Verification items for the finished model (mm, model axes). A direction names the side the tool comes from. Round coordinates to 2 decimals unless told otherwise and drop trailing zeros. Order: outer loops, then holes, each group sorted by start corner. A loop starts at its lowest first (then second) coordinate and runs counter-clockwise, first axis right, second up. Notation, with made-up numbers: (-21, -20.5) -> (-3, -20.5) arc R35 cw to (-3, 17.5) -> close; hole circle Ø2 at (-1, 7). An arc over 180 degrees is marked (long way). Return JSON: item names as keys, results as strings. Group by question number.
1) Section check D-D on z = -291.8. State how many separate pieces and enclosed holes the cut face has, plus the area to 3 significant figures.
2) Tool access check on faces 1 (the flat face through (612.722, -14, -282)), 2 (the cylindrical face through (602.03, -28.09, -291.98)), 3 (the flat face through (597, -20, -292)), 4 (the flat face through (610, -20, -260)), 5 (the flat face through (595.962, -41.363, -306.052)). Record the directions out of +Z, -Z, +X, -X, +Y, -Y that give a thin tool (end or side, any length) a straight path to the whole face; none if there is none.
3) Depth check by flat-ended pin: pin 1 (17 mm diameter, centred on x = 597, z = -287.5, fed in from +Y); pin 2 (13 mm diameter, centred on x = 602.25, y = -36.09, fed in from -Z); pin 3 (4 mm diameter, centred on x = 597.5, y = -37, fed in from +Z); pin 4 (8 mm diameter, centred on y = -11.5, z = -268, fed in from -X). Enter the tip coordinate at first touch or a pass-through.
4) Draft check along X on faces 6 (the flat face through (587.958, -27.433, -291.582)), 7 (the flat face through (607.4, -10, -275)), 8 (the cylindrical face through (609.376, -41.128, -291.618)), 9 (the cylindrical face through (585.32, -9.04, -289.49)). Enter one of: pulls with the +X half, pulls with the -X half, needs draft (parallel to the pull), parting line crosses it, or undercut.
5) Scan lines: L1, parallel to X at y = -3, z = -281; L2, parallel to Y at x = 609.1, z = -260.05; L3, parallel to Z at x = 585.5, y = -22. Record each from-to range of solid material in increasing order.
6) Section check A-A on y = -10. Enter the section's corners in (x, z).
7) Section check C-C on z = -260.05. Enter the section's corners in (x, y).
8) Section check B-B on y = -18. Enter the section's corners in (x, z), plus the area to 3 significant figures.
Autodesk Inventor part; units mm, degrees
ref_plane "YZ Plane" through (0, 0, 0) normal (1, 0, 0) x (0, 1, 0)
ref_plane "XZ Plane" through (0, 0, 0) normal (0, 1, 0) x (-1, 0, 0)
ref_plane "XY Plane" through (0, 0, 0) normal (0, 0, 1) x (1, 0, 0)
ref_plane "Work Plane1" through (0, 0, -304.8) normal (0, 0, 1) x (1, 0, 0)
sketch "Sketch1" plane through (0, 0, -304.8) normal (0, 0, 1) x (1, 0, 0)
  circle A0 centre (602.2484, -36.0888) radius 4
  line L0 (25.4, 0) -> (584.2, 0)
  line L1 (584.2, 0) -> (584.2, -20)
  line L2 (609.6, -20) -> (584.2, -20)
  line L3 (609.6, -20) -> (609.6, 3.175)
  line L4 (0, 3.175) -> (609.6, 3.175)
  line L5 (0, -20) -> (0, 3.175)
  line L6 (25.4, -20) -> (0, -20)
  line L7 (25.4, 0) -> (25.4, -20)
  circle A1 centre (602.2484, -36.0888) radius 8
  line L8 (595.3202, -40.0888) -> (593.5242, -41.8849)
  line L9 (595.3202, -40.0888) -> (597.8602, -40.0888) construction
  arc A2 (591.8233, -35.0767) -> (612.7225, -36.0888) centre (602.2484, -36.0888) ccw
  line L10 (609.6, -20) -> (584.2, -20)
  line L11 (586.9, -20) -> (606.9, -20)
  line L12 (612.7225, -20) -> (609.6, -20)
  line L13 (612.7225, -36.0888) -> (612.7225, -20)
  line L14 (584.2, -20) -> (591.8233, -35.0767)
  point P0 (0, 0)
  dimension "d0" = 16
  dimension "d1" = 2.54
  dimension "d2" = 135
  dimension "d3" = 20
extrude "Extrusion1" add sketch "Sketch1" along normal blind 26 contours L2 L12 L13 A2 L14
sketch "Sketch2" plane through (0, 0, -278.8) normal (0, 0, 1) x (1, 0, 0)
  circle A0 centre (602.2484, -36.0888) radius 8
  line L0 (584.2, -20) -> (591.8233, -35.0767)
  arc A1 (591.8233, -35.0767) -> (612.7225, -36.0888) centre (602.2484, -36.0888) ccw
  line L1 (612.7225, -36.0888) -> (612.7225, -20)
  line L2 (612.7225, -20) -> (584.2, -20)
  circle A2 centre (602.2484, -36.0888) radius 6
  point P0 (0, 0)
  dimension "d7" = 12
extrude "Extrusion2" add sketch "Sketch2" along normal blind 2.54 contours A0 | L2 L1 A1 L0
sketch "Sketch3" plane through (0, 0, -304.8) normal (0, 0, -1) x (-1, 0, 0)
  circle A0 centre (-602.2484, -36.0888) radius 6
  line L0 (-584.2, -20) -> (-591.8233, -35.0767)
  arc A1 (-612.7225, -36.0888) -> (-591.8233, -35.0767) centre (-602.2484, -36.0888) ccw
  line L1 (-612.7225, -36.0888) -> (-612.7225, -20)
  line L2 (-612.7225, -20) -> (-584.2, -20)
  point P0 (0, 0)
extrude "Extrusion3" add sketch "Sketch3" along normal blind 2.54
sketch "Sketch4" plane through (0, 0, -276.26) normal (0, 0, 1) x (1, 0, 0)
  circle A0 centre (602.2484, -36.0888) radius 6
  line L0 (584.2, -20) -> (591.8233, -35.0767)
  arc A1 (591.8233, -35.0767) -> (612.7225, -36.0888) centre (602.2484, -36.0888) ccw
  line L1 (612.7225, -36.0888) -> (612.7225, -20)
  line L2 (612.7225, -20) -> (584.2, -20)
  line L3 (602.2484, -36.0888) -> (610.272, -42.8214)
  arc A2 (591.8233, -35.0767) -> (612.7225, -36.0888) centre (602.2484, -36.0888) ccw
  line L4 (602.2484, -36.0888) -> (612.7225, -36.0888) construction
  circle A3 centre (602.2484, -36.0888) radius 6
  line L5 (602.2484, -36.0888) -> (594.2248, -42.8214)
  line L6 (602.2484, -36.0888) -> (612.7225, -36.0888) construction
  arc A4 (594.2248, -42.8214) -> (610.272, -42.8214) centre (602.2484, -36.0888) ccw
  line L7 (602.2484, -36.0888) -> (594.2248, -42.8214)
  line L8 (602.2484, -36.0888) -> (610.272, -42.8214)
  point P0 (0, 0)
  dimension "d12" = 40
  dimension "d13" = 140
extrude "Extrusion4" cut sketch "Sketch4" against normal blind 39.0525 contours L5 L3 A0 | A0 L3 A1 L5 picked at (604.1466, -39.5744)
fillet "Fillet1" radius 3.175 2 edges at (596.1201, -41.2311, -291.8) (608.3768, -41.2311, -291.8)
sketch "Sketch5" plane through (0, 0, -276.26) normal (0, 0, 1) x (1, 0, 0)
  point P0 (0, 0)
sketch "Sketch6" plane through (0, 0, -307.34) normal (0, 0, -1) x (-1, 0, 0)
  point P0 (0, 0)
sketch "Sketch7" plane through (0, 0, -307.34) normal (0, 0, -1) x (-1, 0, 0)
  line L0 (-25.4, 0) -> (-584.2, 0)
  line L1 (-584.2, 0) -> (-584.2, -20)
  line L2 (-609.6, -20) -> (-584.2, -20)
  line L3 (-609.6, -20) -> (-609.6, 3.175)
  line L4 (0, 3.175) -> (-609.6, 3.175)
  line L5 (0, -20) -> (0, 3.175)
  line L6 (-25.4, -20) -> (0, -20)
  line L7 (-25.4, 0) -> (-25.4, -20)
  line L8 (-606.8447, -39.9455) -> (-610.272, -42.8214)
  arc A0 (-612.7225, -36.0888) -> (-610.272, -42.8214) centre (-602.2484, -36.0888) ccw
  line L9 (-612.7225, -36.0888) -> (-612.7225, -20)
  line L10 (-612.7225, -20) -> (-584.2, -20)
  line L11 (-584.2, -20) -> (-591.8233, -35.0767)
  arc A1 (-594.2248, -42.8214) -> (-591.8233, -35.0767) centre (-602.2484, -36.0888) ccw
  line L12 (-594.2248, -42.8214) -> (-597.6521, -39.9455)
  arc A2 (-597.6521, -39.9455) -> (-606.8447, -39.9455) centre (-602.2484, -36.0888) ccw
  line L13 (-586.4, 0) -> (-586.4, -20)
  line L14 (-607.4, -20) -> (-607.4, 0)
  line L15 (-586.4, 0) -> (-584.2, 0)
  line L16 (-584.2, 0) -> (-584.2, -20)
  line L17 (-584.2, -20) -> (-586.4, -20)
  line L18 (-586.4, 0) -> (-586.4, -20)
  line L19 (-607.4, 0) -> (-609.6, 0)
  line L20 (-609.6, 0) -> (-609.6, -20)
  line L21 (-609.6, -20) -> (-607.4, -20)
  point P0 (0, 0)
  dimension "d17" = 21
  dimension "d18" = 20
extrude "Extrusion5" add sketch "Sketch7" against normal up to surface (31.08 mm away) contours L1 L2 L13 L15 | L2 L3 L19 L14
sketch "Sketch8" plane through (609.6, -20, -307.34) normal (1, 0, 0) x (0, 0, -1)
  line L0 (-31.08, 20) -> (-31.08, 0)
  line L1 (0, 0) -> (-31.08, 0)
  line L2 (0, 20) -> (0, 0)
  line L3 (0, 20) -> (-31.08, 20)
  point P0 (-307.34, 20)
extrude "Extrusion6" add sketch "Sketch8" along normal up to surface (3.1225 mm away)
sketch "Sketch9" plane through (612.7225, -36.0888, -276.26) normal (1, 0, 0) x (0, 0, -1)
  line L0 (0, -3.8567) -> (0, -6.7326)
  line L1 (0, -6.7326) -> (0, 0)
  line L2 (0, 0) -> (0, 36.0888)
  line L3 (0, 16.0888) -> (0, 36.0888)
  line L4 (0, 36.0888) -> (0, 16.0888)
  line L5 (0, 16.0888) -> (0, 36.0888)
  line L6 (0, 16.0888) -> (0, 1.0121)
  line L7 (0, 1.0121) -> (0, -6.7326)
  line L8 (0, -6.7326) -> (0, -3.8567)
  line L9 (0, -3.8567) -> (0, -3.8567)
  line L10 (31.08, 16.0888) -> (0, 16.0888)
  line L11 (31.08, 16.0888) -> (-32.42, 16.0888)
  line L12 (-32.42, 16.0888) -> (-32.42, 36.0888)
  line L13 (-32.42, 36.0888) -> (31.08, 36.0888)
  line L14 (31.08, 36.0888) -> (31.08, 16.0888)
  point P0 (-276.26, 36.0888)
  dimension "d23" = 63.5
  dimension "d24" = 20
extrude "Extrusion7" add sketch "Sketch9" against normal up to surface (5.3225 mm away)
sketch "Sketch10" plane through (607.4, -20, -307.34) normal (-1, 0, 0) x (0, 0, 1)
  line L0 (31.08, -16.0888) -> (31.08, 0)
  line L1 (0, -16.0888) -> (31.08, -16.0888)
  line L2 (0, 20) -> (0, -16.0888)
  line L3 (63.5, 20) -> (0, 20)
  line L4 (63.5, 20) -> (63.5, 0)
  line L5 (63.5, 0) -> (31.08, 0)
  circle A0 centre (47.29, 10) radius 2.5
  circle A1 centre (15.54, 10) radius 2.5
  point P0 (307.34, 20)
  dimension "d27" = 5
  dimension "d28" = 5
extrude "Extrusion8" cut sketch "Sketch10" along normal mid plane 254 contours A0 | A1
properties part number "Bed Slider"
Check result:
{
 "1": {"separate pieces": "3", "enclosed holes": "0", "area": "435 mm^2"},
 "2": {"face 1": "+Z, -Z, +X, +Y, -Y", "face 2": "none", "face 3": "+Z, -Z, +Y", "face 4": "+Z, +X, -X, -Y", "face 5": "+Z, -Z, -Y"},
 "3": {"pin 1": "y = -20", "pin 2": "z = -307.34", "pin 3": "z = -276.26", "pin 4": "x = 607.4"},
 "4": {"face 6": "pulls with the -X half", "face 7": "undercut", "face 8": "undercut", "face 9": "needs draft"},
 "5": {"L1": "584.2 to 586.4, 607.4 to 612.72", "L2": "-20 to -12.5, -7.5 to 0", "L3": "-307.34 to -276.26"},
 "6": {"outline": "(584.2, -307.34) -> (586.4, -307.34) -> (586.4, -294.3) -> (584.2, -294.3) -> close; (584.2, -289.3) -> (586.4, -289.3) -> (586.4, -276.26) -> (584.2, -276.26) -> close; (607.4, -307.34) -> (612.72, -307.34) -> (612.72, -294.3) -> (607.4, -294.3) -> close; (607.4, -289.3) -> (612.72, -289.3) -> (612.72, -262.55) -> (607.4, -262.55) -> close; (607.4, -257.55) -> (612.72, -257.55) -> (612.72, -243.84) -> (607.4, -243.84) -> close"},
 "7": {"outline": "(607.4, -20) -> (612.72, -20) -> (612.72, -12.5) -> (607.4, -12.5) -> close; (607.4, -7.5) -> (612.72, -7.5) -> (612.72, 0) -> (607.4, 0) -> close"},
 "8": {"outline": "(584.2, -307.34) -> (586.4, -307.34) -> (586.4, -276.26) -> (584.2, -276.26) -> close; (607.4, -307.34) -> (612.72, -307.34) -> (612.72, -243.84) -> (607.4, -243.84) -> close", "area": "406 mm^2"}
}
